The model under review builds one solid part; all positions refer to its coordinate system, in mm. A direction names the side the tool comes from. Coordinates: 2 decimals unless noted, no trailing zeros. Write each loop counter-clockwise with the first axis right and the second up, starting at its lowest first coordinate (ties: lowest second). Pieces come first, ordered by that corner, then holes.
1) Mouldability with a two-part tool opening along Z and no side actions: class faces 1 (the cylindrical face through (-26.84, -46.22, -31.01)), 2 (the cylindrical face through (-26.84, 18.38, -30.22)), 3 (the cylindrical face through (-28, -53, 39)), 4 (the cylindrical face through (-28, -54, -38)) as released by +Z, released by -Z, zero draft, split by the parting line, or undercut.
2) Add section B-B, the plane x = -38. State the section outline as (y, z) points.
3) For P1, Ø2.5, axis at x = 15.5, y = 4, coming from the -Z side; P2, Ø4.5, axis at x = 8.5, z = -0.5, coming from the +Y side; P3, Ø7, axis at y = 18.25, z = -33.22, coming from the +X side, all flat-tipped, find the tip position at first contact; note any pin that passes through.
4) Add section D-D, the plane x = 18. State the section outline as (y, z) points, then the cut area to 3 significant figures.
5) Machinability: for faces 5 (the cylindrical face through (-3.5, 12.4, 6.5)), 6 (the flat face through (-46.3, -14, -1)), 7 (the cylindrical face through (-26.84, 18.382, 36.215)), 8 (the flat face through (15, 2.5, 0)), which of the approach directions +Z, -Z, +X, -X, +Y, -Y give a long, thin tool a straight path to every point of the face, cutting with its end or side? Answer none if there is none.
6) Add section A-A, the plane y = 18.25. State the section outline as (x, z) points.
7) Add section C-C, the plane z = -12. State the section outline as (x, y) points, then the cut area to 3 significant figures.
8) For line 1 (Z direction, x = -20, y = 18); line 2 (Z direction, x = -47.5, y = -15); line 3 (X direction, y = -41.5, z = 11.5), list the stretches that pass through material, from the lowest coordinate up.
from build123d import *

# Parameters (mm, degrees)
SKETCH1_W           = 80
SKETCH1_H           = 80
BOSS_EXTRUDE1_DEPTH = 44.3
SKETCH2_R           = 3
CUT_EXTRUDE1_DEPTH  = 82.1633538
FILLET1_R           = 5
FILLET2_R           = 1
FILLET3_R           = 1
CUT_EXTRUDE2_DEPTH  = 25
FILLET4_R           = 2
SKETCH5_W           = 3
SKETCH5_H           = 36.5


with BuildPart() as part:
    # Sketch1 → Boss-Extrude1 (new body)
    with BuildSketch(Plane(origin=(-5, 0, 0), x_dir=(0, 0, -1), z_dir=(1, 0, 0))):
        with Locations((0, -15)):
            Rectangle(SKETCH1_W, SKETCH1_H)
    extrude(amount=-BOSS_EXTRUDE1_DEPTH)

    # Sketch2 → Cut-Extrude1 (cut, through all)
    with BuildSketch(Plane(origin=(-5, 0, 0), x_dir=(0, 0, -1), z_dir=(1, 0, 0))):
        with Locations((-33.218029743, 18.25)):
            Circle(SKETCH2_R)
        with Locations((33.218029743, 18.25)):
            Circle(SKETCH2_R)
        with Locations((33.218029743, -48.25)):
            Circle(SKETCH2_R)
        with Locations((-33.218029743, -48.25)):
            Circle(SKETCH2_R)
    extrude(amount=-CUT_EXTRUDE1_DEPTH, mode=Mode.SUBTRACT)

    # Fillet1
    fillet1_edges = [part.edges().sort_by_distance(p)[0] for p in [
        (-27.15, 25, 40),
        (-27.15, 25, -40),
        (-27.15, -55, -40),
        (-27.15, -55, 40),
    ]]
    fillet(fillet1_edges, radius=FILLET1_R)

    # Fillet2
    fillet2_edges = [part.edges().sort_by_distance(p)[0] for p in [
        (-5, -55, 0),
        (-5, -15, 40),
        (-5, -15, -40),
        (-5, 25, 0),
        (-5, 23.535533906, -38.535533906),
        (-5, 23.535533906, 38.535533906),
        (-5, -53.535533906, 38.535533906),
        (-5, -53.535533906, -38.535533906),
    ]]
    fillet(fillet2_edges, radius=FILLET2_R)

    # Sketch3 → Revolve1 (revolve)
    with BuildSketch(Plane.XY, mode=Mode.PRIVATE) as revolve1_sk:
        with BuildLine():
            Line((-5, 14), (-2, 14))
            Line((-2, 14), (-2, 6))
            Line((-2, 6), (0, 6))
            ThreePointArc((0, 6), (0.732050808, 5.267949192), (1.732050808, 5))
            Line((1.732050808, 5), (27, 5))
            Line((27, 5), (27, 0))
            Line((27, 0), (-5, 0))
            Line((-5, 0), (-5, 14))
        make_face()
    revolve(revolve1_sk.sketch.rotate(Axis((-5, 0, 0), (1, 0, 0)), 90), axis=Axis((-5, 0, 0), (1, 0, 0)))

    # Fillet3
    fillet3_edges = [part.edges().sort_by_distance(p)[0] for p in [
        (27, 0, -5),
    ]]
    fillet(fillet3_edges, radius=FILLET3_R)

    # Sketch4 → Cut-Extrude2 (cut)
    with BuildSketch(Plane(origin=(27, 0, 0), x_dir=(0, 0, -1), z_dir=(1, 0, 0))):
        with BuildLine():
            Line((2, 4.582575695), (2, 2.5))
            Line((2, 2.5), (-2, 2.5))
            Line((-2, 2.5), (-2, 4.582575695))
            ThreePointArc((-2, 4.582575695), (0, 5), (2, 4.582575695))
        make_face()
    extrude(amount=-CUT_EXTRUDE2_DEPTH, mode=Mode.SUBTRACT)

    # Fillet4
    fillet4_edges = [part.edges().sort_by_distance(p)[0] for p in [
        (2, 3.541287847, -2),
        (2, 3.541287847, 2),
    ]]
    fillet(fillet4_edges, radius=FILLET4_R - 0.0001)  # a hair under: the kernel refuses the full size

    # Sketch5 → Cut-Revolve1 (revolve, cut)
    with BuildSketch(Plane.XY):
        with Locations((-47.8, 3.25)):
            Rectangle(SKETCH5_W, SKETCH5_H)
    revolve(axis=Axis((-46.3, -15, 0), (-1, 0, 0)), mode=Mode.SUBTRACT)


solid = part.part
Geometry results:
1. face 1: undercut
1. face 2: undercut
1. face 3: released by +Z
1. face 4: released by -Z
2. outline: (-55, -35) arc R5 ccw to (-50, -40) - (20, -40) arc R5 ccw to (25, -35) - (25, 35) arc R5 ccw to (20, 40) - (-50, 40) arc R5 ccw to (-55, 35) - close; hole circle Ø6 at (-48.25, -33.22); hole circle Ø6 at (-48.25, 33.22); hole circle Ø6 at (18.25, -33.22); hole circle Ø6 at (18.25, 33.22)
3. P1: stops at z = -4.18
3. P2: stops at y = 4.58
3. P3: stops at x = -5
4. outline: (2.5, -2) - (2.5, 2) - (4.58, 2) arc R5 ccw (long way) to (4.58, -2) - close
4. area: 69.1 mm2
5. face 5: +X
5. face 6: -X
5. face 7: +X, -X
5. face 8: +X, +Y
6. outline: (-49.3, -40) - (-6, -40) arc R1 ccw to (-5, -39) - (-5, -36.22) - (-49.3, -36.22) - close; (-49.3, -30.22) - (-5, -30.22) - (-5, 30.22) - (-49.3, 30.22) - (-49.3, 15.06) - (-46.3, 15.06) - (-46.3, -15.06) - (-49.3, -15.06) - close; (-49.3, 36.22) - (-5, 36.22) - (-5, 39) arc R1 ccw to (-6, 40) - (-49.3, 40) - close
7. outline: (-49.3, -55) - (-6, -55) arc R1 ccw to (-5, -54) - (-5, -7.21) - (-2, -7.21) - (-2, 7.21) - (-5, 7.21) - (-5, 24) arc R1 ccw to (-6, 25) - (-49.3, 25) - (-49.3, 19.47) - (-46.3, 19.47) - (-46.3, -49.47) - (-49.3, -49.47) - close
7. area: 3,380 mm2
8. line 1: z = -40 to -36.21, -30.23 to 30.23, 36.21 to 40
8. line 2: z = -40 to -36.5, 36.5 to 40
8. line 3: x = -46.3 to -5
